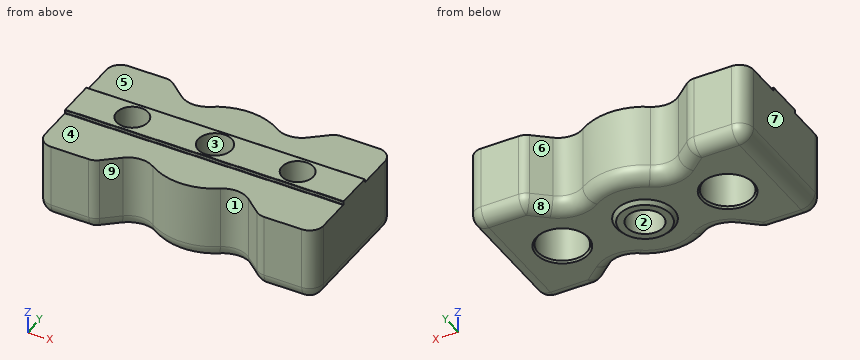
Autodesk Inventor part; units mm, degrees
ref_plane "YZ Plane" through (0, 0, 0) normal (1, 0, 0) x (0, 1, 0)
ref_plane "XZ Plane" through (0, 0, 0) normal (0, 1, 0) x (-1, 0, 0)
ref_plane "XY Plane" through (0, 0, 0) normal (0, 0, 1) x (1, 0, 0)
sketch "Sketch1" plane through (0, 0, 0) normal (0, 0, 1) x (1, 0, 0)
  line L0 (-40, 19.775) -> (40, 19.775)
  line L1 (40, 19.775) -> (40, -19.775)
  line L2 (40, -19.775) -> (-40, -19.775)
  line L3 (-40, -19.775) -> (-40, 19.775)
  line L4 (-40, 19.775) -> (40, -19.775) construction
  line L5 (40, 19.775) -> (-40, -19.775) construction
  line L6 (40, -5.5) -> (-40, -5.5)
  line L7 (-40, -5.5) -> (-40, 5.5)
  line L8 (-40, 5.5) -> (40, 5.5)
  line L9 (40, 5.5) -> (40, -5.5)
  line L10 (40, -5.5) -> (-40, 5.5) construction
  line L11 (-40, -5.5) -> (40, 5.5) construction
  line L12 (23.75, 0) -> (-23.75, 0)
  circle A0 centre (-23.75, 0) radius 4.5
  circle A1 centre (23.75, 0) radius 4.5
  circle A2 centre (0, 0) radius 8
  point P0 (-40, 5.5)
  point P1 (-40, -5.5)
  point P2 (40, -5.5)
  point P3 (-5.8095, -5.5)
  point P4 (5.8095, -5.5)
  point P5 (5.8095, 5.5)
  point P6 (-5.8095, 5.5)
  dimension "d0" = 80
  dimension "d1" = 39.55
  dimension "d3" = 11
  dimension "d9" = 80
  dimension "d10" = 47.5
  dimension "d11" = 9
  dimension "d12" = 9
  dimension "d13" = 19.775
  dimension "d14" = 14.275
  dimension "d15" = 16
extrude "Extrusion1" add sketch "Sketch1" along normal blind 1 contours L8 A2 L6 L3 | L1 L6 A2 L8 | L8 A2 L12 | A2 L12 L6
extrude "Extrusion2" add sketch "Sketch1" against normal blind 6
fillet "Fillet1" radius 0.2 4 edges at (0, 5.5, 0) (0, 5.5, 1) (0, -5.5, 1) (0, -5.5, 0)
sketch "Sketch2" plane through (0, 0, -6) normal (0, 0, -1) x (-1, 0, 0)
  circle A0 centre (23.75, 0) radius 4.5
  circle A1 centre (-23.75, 0) radius 4.5
  circle A2 centre (23.75, 0) radius 7
  circle A3 centre (-23.75, 0) radius 7
  line L0 (-40, -19.775) -> (40, -19.775)
  line L1 (-40, 19.775) -> (-40, -19.775)
  line L2 (40, 19.775) -> (-40, 19.775)
  line L3 (40, -19.775) -> (40, 19.775)
  point P0 (0, 0)
  dimension "d16" = 14
  dimension "d17" = 14
extrude "Extrusion3" add sketch "Sketch2" along normal blind 16 contours L1 L2 L3 L0
sketch "Sketch3" plane through (0, 0, -22) normal (0, 0, -1) x (-1, 0, 0)
  circle A0 centre (0, 0) radius 5.15
  dimension "d21" = 10.3
extrude "Extrusion4" cut sketch "Sketch3" against normal blind 10
sketch "Sketch4" plane through (0, 0, -22) normal (0, 0, -1) x (-1, 0, 0)
  circle A0 centre (0, 0) radius 5.15
  circle A1 centre (0, 0) radius 7.25
  dimension "d24" = 14.5
extrude "Extrusion5" add sketch "Sketch4" along normal blind 1
chamfer "Chamfer1" distance 1 distance2 1 1 edges at (7.25, 0, -22) measured on face at (-0.2913, -15.5824, -22)
sketch "Sketch5" plane through (0, 0, -12) normal (0, 0, -1) x (-1, 0, 0)
  circle A0 centre (0, 0) radius 4.8
  dimension "d30" = 9.6
extrude "Extrusion6" cut sketch "Sketch5" against normal blind 20
sketch "Sketch6" plane through (0, 0, -22) normal (0, 0, -1) x (-1, 0, 0)
  circle A0 centre (0, 0) radius 17.5
  circle A1 centre (23.75, 0) radius 7
  circle A2 centre (-23.75, 0) radius 7
  line L0 (40, -19.775) -> (40, 19.775)
  line L1 (40, 19.775) -> (-40, 19.775)
  line L2 (-40, 19.775) -> (-40, -19.775)
  line L3 (-40, -19.775) -> (40, -19.775)
  circle A3 centre (0, 0) radius 8.25
  line L4 (-23.75, 0) -> (-23.75, 19.775)
  line L5 (13.4485, 11.1977) -> (23.75, 19.775)
  line L6 (-40, 19.775) -> (40, 19.775)
  line L7 (-23.75, 19.775) -> (-13.4485, 11.1977)
  dimension "d33" = 35
extrude "Extrusion7" cut sketch "Sketch6" against normal through all contours A0 L7 L1 L5
mirror "Mirror1" about plane through (0, 0, 0) normal (0, 1, 0) of "Extrusion7"
fillet "Fillet3" radius 7 4 edges at (13.4485, 11.1977, -11) (-13.4485, 11.1977, -11) (13.4485, -11.1977, -11) (-13.4485, -11.1977, -11)
fillet "Fillet4" radius 4 8 edges at (23.75, -19.775, -11) (40, -19.775, -11) (40, 19.775, -11) (23.75, 19.775, -11) (-23.75, 19.775, -11) (-40, 19.775, -11) (-40, -19.775, -11) (-23.75, -19.775, -11)
fillet "Fillet5" radius 4 24 edges at (38.8284, 18.6034, -22) (40, 0, -22) (38.8284, -18.6034, -22) (30.5986, -19.775, -22) (23.8363, -19.5364, -22) (20.3404, -16.9361, -22) (13.9404, -13.4128, -22) (0, -17.5, -22) (-13.9404, -13.4128, -22) (-20.3404, -16.9361, -22) (-23.8363, -19.5364, -22) (-30.5986, -19.775, -22) (-38.8284, -18.6034, -22) (-40, 0, -22) (-38.8284, 18.6034, -22) (-30.5986, 19.775, -22) (-23.8363, 19.5364, -22) (-20.3404, 16.9361, -22) (-13.9404, 13.4128, -22) (0, 17.5, -22) (13.9404, 13.4128, -22) (20.3404, 16.9361, -22) (23.8363, 19.5364, -22) (30.5986, 19.775, -22)
chamfer "Chamfer2" distance 0.5 angle 45 2 edges at (-16.75, 0, -22) (30.75, 0, -22)
equation "\"d9\" = d0"
properties part number "Base_Mount_Pedals"
The listing builds one solid part. Answer for the finished solid, in the listing's coordinates (mm). Face numbers are marked on the shaded views. A direction names the side the tool comes from. Give positions to 0.01 mm unless a question says otherwise; leave off trailing zeros. Write each loop counter-clockwise with the first axis right and the second up, starting at its lowest first coordinate (ties: lowest second). Pieces come first, ordered by that corner, then holes. Notation, with made-up numbers: (29.25, 5) - (47.25, 5) arc R9 ccw to (47.25, 17) - close; hole circle Ø10 at (-11, -14). An arc over 180 degrees is marked (long way). One line per question, with ' | ' between items. Start each with the question number.
1. Section D-D, the plane y = 0 is taken. Count the separate pieces of the cut face and the enclosed holes in it, then the cut area to 3 significant figures.
2. Determine the mould class of the marked faces 1, 2, 3 and 4 for opening direction Y: +Y half, -Y half, draft (parallel to the pull), parting line (faces both ways), or undercut.
3. Section B-B, the plane z = -10 is taken. Determine the outline of the cut face in (x, y) (3 decimals).
4. Straight lines are drawn through the part: line 1 (Y direction, x = 0, z = -8.25); line 2 (X direction, y = 15, z = -19.25); line 3 (Y direction, x = 0, z = -15). For each, find the intervals that lie inside material, in ascending order.
5. Section C-C, the plane z = -3.5 is taken. Determine the outline of the cut face in (x, y) (3 decimals).
6. Given P1, Ø1, axis at x = -20.5, z = -2.5, coming from the +Y side; P2, Ø11, axis at x = -27, y = -1, coming from the -Z side; P3, Ø5, axis at x = 17, y = -15.5, coming from the -Z side, each flat-ended and moving along its own axis, determine where each tip first touches the part or whether it passes through.
7. For the marked faces 5, 6, 7, 8 and 9, determine the directions among +Z, -Z, +X, -X, +Y, -Y from which every point of the face is accessible in a straight line to the end or side of a thin tool.
Result:
1) separate pieces: 4 | enclosed holes: 0 | area: 1,040 mm2
2) face 1: -Y half | face 2: undercut | face 3: undercut | face 4: draft
3) outline: (-40, -15.775) arc R4 ccw to (-36, -19.775) - (-25.197, -19.775) arc R4 ccw to (-22.638, -18.849) - (-18.043, -15.023) arc R7 cw to (-9.689, -14.573) arc R17.5 ccw to (9.689, -14.573) arc R7 cw to (18.043, -15.023) - (22.638, -18.849) arc R4 ccw to (25.197, -19.775) - (36, -19.775) arc R4 ccw to (40, -15.775) - (40, 15.775) arc R4 ccw to (36, 19.775) - (25.197, 19.775) arc R4 ccw to (22.638, 18.849) - (18.043, 15.023) arc R7 cw to (9.689, 14.573) arc R17.5 ccw to (-9.689, 14.573) arc R7 cw to (-18.043, 15.023) - (-22.638, 18.849) arc R4 ccw to (-25.197, 19.775) - (-36, 19.775) arc R4 ccw to (-40, 15.775) - close; hole circle Ø14 at (-23.75, 0); hole circle Ø9.6 at (0, 0); hole circle Ø14 at (23.75, 0)
4) line 1: y = -17.5 to -4.8, 4.8 to 17.5 | line 2: x = -39.8 to -18.33, -8.62 to 8.62, 18.33 to 39.8 | line 3: y = -17.5 to -5.15, 5.15 to 17.5
5) outline: (-40, -15.775) arc R4 ccw to (-36, -19.775) - (-25.197, -19.775) arc R4 ccw to (-22.638, -18.849) - (-18.043, -15.023) arc R7 cw to (-9.689, -14.573) arc R17.5 ccw to (9.689, -14.573) arc R7 cw to (18.043, -15.023) - (22.638, -18.849) arc R4 ccw to (25.197, -19.775) - (36, -19.775) arc R4 ccw to (40, -15.775) - (40, 15.775) arc R4 ccw to (36, 19.775) - (25.197, 19.775) arc R4 ccw to (22.638, 18.849) - (18.043, 15.023) arc R7 cw to (9.689, 14.573) arc R17.5 ccw to (-9.689, 14.573) arc R7 cw to (-18.043, 15.023) - (-22.638, 18.849) arc R4 ccw to (-25.197, 19.775) - (-36, 19.775) arc R4 ccw to (-40, 15.775) - close; hole circle Ø9 at (-23.75, 0); hole circle Ø9.6 at (0, 0); hole circle Ø9 at (23.75, 0)
6) P1: stops at y = 17.49 | P2: stops at z = -22 | P3: stops at z = -21.11
7) face 5: +Z, +X, -X, +Y | face 6: +Z, -Z, +Y | face 7: +Z, -Z, -X, +Y, -Y | face 8: -Z, +Y | face 9: +Z, -Z, -Y
